from build123d import *

# Parameters (mm, degrees)
SKETCH004_R      = 2.7
PAD003_DEPTH     = 8.2
SKETCH005_R      = 5
POCKET001_DEPTH  = 2
CHAMFER002_SIZE  = 3
CHAMFER003_SIZE2 = 55
CHAMFER003_SIZE  = 6
FILLET_R         = 200
CHAMFER004_SIZE  = 3


with BuildPart() as part:
    # Sketch004 (on XY_Plane003 of Origin006) → Pad003 (new body)
    with BuildSketch(Plane.XY):
        Polygon((268.465729, 19.911931), (182.088478, 28.044908), (179.447869, 0), (266.590892, 0), align=None)
        with Locations((196.085008, 16.682815)):
            Circle(SKETCH004_R, mode=Mode.SUBTRACT)
    extrude(amount=PAD003_DEPTH)

    # Sketch005 (on Face7 of Pad003) → Pocket001 (cut)
    with BuildSketch(Plane.XY.offset(8.2)):
        with Locations((196.085008, 16.682815)):
            Circle(SKETCH005_R)
    extrude(amount=-POCKET001_DEPTH, mode=Mode.SUBTRACT)

    # Chamfer002
    chamfer002_edges = [part.edges().sort_by_distance(p)[0] for p in [
        (182.088478, 28.044908, 4.1),
    ]]
    chamfer(chamfer002_edges, length=CHAMFER002_SIZE)

    # Chamfer003
    chamfer003_edges = [part.edges().sort_by_distance(p)[0] for p in [
        (267.52831, 9.955965, 8.2),
    ]]
    chamfer003_side = part.faces().sort_by_distance((267.52831, 9.955965, 4.1))[0]
    chamfer(chamfer003_edges, length=CHAMFER003_SIZE, length2=CHAMFER003_SIZE2, reference=chamfer003_side)

    # Fillet
    fillet_edges = [part.edges().sort_by_distance(p)[0] for p in [
        (212.527775, 12.533867, 8.2),
    ]]
    fillet(fillet_edges, radius=FILLET_R)

    # Chamfer004
    chamfer004_edges = [part.edges().sort_by_distance(p)[0] for p in [
        (268.465729, 19.911931, 1.1),
    ]]
    chamfer(chamfer004_edges, length=CHAMFER004_SIZE)

    # Mirrored001: part across face of Chamfer004


with BuildPart() as part_1:
    add(part.part)
    add(part.part.mirror(Plane(origin=(215.438972, 0, 3.448187), x_dir=(1, 0, 0), z_dir=(0, -1, 0))))


solid = part_1.part
Source: CAD feature listing. Evaluate the final solid. Frame: model axes, mm. A direction names the side the tool comes from. Give positions to 0.01 mm unless a question says otherwise; leave off trailing zeros. Write each loop counter-clockwise with the first axis right and the second up, starting at its lowest first coordinate (ties: lowest second). Pieces come first, ordered by that corner, then holes. Notation, with made-up numbers: (2, 38) - (10, 38) arc R18 ccw to (10, 60) - close; hole circle Ø6 at (-6.75, 44.5). An arc over 180 degrees is marked (long way). Write item = value, one per line. Start each with the question number.
Q1. Cut plane B-B, the plane x = 258.5. Return loops of the section in (y, z), then the cut area to 3 significant figures.
Q2. Reachability of faces 4 (the flat face through (267.377, 8.344, 1.085)), 5 (the flat face through (216.906, 24.767, 3.131)), 6 (the cylindrical face through (212.6, -12.2, 7.9)), 7 (the flat face through (223, 0, 0)), 8 (the cylindrical face through (198.77, -20.9, 7.21)) from +Z, -Z, +X, -X, +Y, -Y: full face, straight path, thin tool, end or side. Return the list, or none.
Q3. Draft query along Y for faces 1 (the flat face through (180.644, -12.704, 4.043)), 2 (the flat face through (266.85, 18.54, 1.25)), 3 (the flat face through (267.377, -8.344, 1.085)). Return one class per face: +Y half, -Y half, draft (parallel to the pull), parting line (faces both ways), or undercut.
Q4. Cut plane A-A, the plane z = 4.5. Return loops of the section in (x, y) (3 decimals).
Q5. Material intervals for probe 1 along Z at (x, y) = (222.5, -1.5); probe 2 along Z at (x, y) = (194.5, 14); probe 3 along X at (y, z) = (10, 0.5), sorted ascending.
Q6. Cut plane C-C, the plane x = 228.5. Return loops of the section in (y, z), then the cut area to 3 significant figures.
Q7. Pin query (flat end, axial travel): pin 1 Ø1 at (x, y) = (208, 19.5) entering from +Z; pin 2 Ø5 at (x, y) = (196.09, -16.68) entering from -Z; pin 3 Ø2 at (x, y) = (223, -8.5) entering from +Z; pin 4 Ø1 at (x, z) = (221, 2) entering from -Y. Return the tip coordinate at first contact, or that it passes through.
Computed values:
q1.outline = (-20.85, 0) - (20.85, 0) - (20.85, 3.29) - (0, 3.08) - (-20.85, 3.29) - close
q1.area = 133 mm²
q2.face_4 = +Z, -Z, +X
q2.face_5 = +Z, -Z, +X, +Y
q2.face_6 = +Z, +X
q2.face_7 = -Z, +X, -X, +Y, -Y
q2.face_8 = +Z
q3.face_1 = -Y half
q3.face_2 = +Y half
q3.face_3 = undercut
q4.outline = (179.448, 0) - (181.807, -25.058) - (185.075, -27.764) - (247.475, -21.888) - (245.414, 0) - (247.475, 21.888) - (185.075, 27.764) - (181.807, 25.058) - close; hole circle Ø5.4 at (196.085, -16.683); hole circle Ø5.4 at (196.085, 16.683)
q5.probe_1 = 0 to 7
q5.probe_2 = 0 to 6.2
q5.probe_3 = 180.39 to 267.53
q6.outline = (-23.67, 0) - (23.67, 0) - (23.67, 6.58) - (0, 6.34) - (-23.67, 6.58) - close
q6.area = 306 mm²
q7.pin_1 = 8.13
q7.pin_2 = through
q7.pin_3 = 7.13
q7.pin_4 = -24.43
